Source: CAD feature listing. Evaluate the final solid. Frame: model axes, mm. A direction names the side the tool comes from. Give positions to 0.01 mm unless a question says otherwise; leave off trailing zeros. Loops run counter-clockwise (first coordinate to the right, second up) from the corner with the lowest first, then second, coordinate; pieces in that order, holes last. Notation, with made-up numbers: M -15,72 L 6,72 A24 cw 6,96 Z; hole C 58,-22 d9. An arc over 180 degrees is marked long. Answer in a Markdown table with one row per item.
```python
from build123d import *

# Parameters (mm, degrees)
SKETCH1_W           = 220
SKETCH1_H           = 130
BOSS_EXTRUDE1_DEPTH = 6
SKETCH2_W           = 90
SKETCH2_H           = 30
CUT_EXTRUDE1_DEPTH  = 128.910124697
FILLET1_R           = 15
SKETCH3_W           = 30
SKETCH3_H           = 6.2
BOSS_EXTRUDE2_DEPTH = 6


with BuildPart() as part:
    # Sketch1 → Boss-Extrude1 (new body)
    with BuildSketch(Plane(origin=(0, 0, 0), x_dir=(1, 0, 0), z_dir=(0, 1, 0))):
        Rectangle(SKETCH1_W, SKETCH1_H)
    extrude(amount=BOSS_EXTRUDE1_DEPTH)

    # Sketch2 → Cut-Extrude1 (cut, through all)
    with BuildSketch(Plane(origin=(0, 6, 0), x_dir=(1, 0, 0), z_dir=(0, 1, 0))):
        with Locations((-35, -50)):
            Rectangle(SKETCH2_W, SKETCH2_H)
        with Locations((-35, 50)):
            Rectangle(SKETCH2_W, SKETCH2_H)
    extrude(amount=-CUT_EXTRUDE1_DEPTH, mode=Mode.SUBTRACT)

    # Fillet1
    fillet1_edges = [part.edges().sort_by_distance(p)[0] for p in [
        (-80, 3, 35),
        (10, 3, 35),
        (-80, 3, -35),
        (10, 3, -35),
    ]]
    fillet(fillet1_edges, radius=FILLET1_R)

    # Sketch3 → Boss-Extrude2 (add)
    with BuildSketch(Plane(origin=(0, 6, 0), x_dir=(1, 0, 0), z_dir=(0, 1, 0))):
        with Locations((-95, 68.1)):
            Rectangle(SKETCH3_W, SKETCH3_H)
        with Locations((-95, -68.1)):
            Rectangle(SKETCH3_W, SKETCH3_H)
    extrude(amount=-BOSS_EXTRUDE2_DEPTH)


solid = part.part
```
Q1. Reachability of faces 1 (the flat face through (59, 3, 65)), 2 (the flat face through (-80, 3, 61)), 3 (the cylindrical face through (5.49, 2.96, -39.28)), 4 (the flat face through (59, 3, -65)) from +Z, -Z, +X, -X, +Y, -Y: full face, straight path, thin tool, end or side. Return the list, or none.
Values follow:
| item | result |
|---|---|
| face 1 | +Z, +X, +Y, -Y |
| face 2 | +Z, +Y, -Y |
| face 3 | -Z, +Y, -Y |
| face 4 | -Z, +X, +Y, -Y |
Q2. Contact query for flat-ended pins moving along their axis: pin 1 Ø1.8 at (x, y) = (45, 3.5) entering from +Z; pin 2 Ø1 at (x, y) = (36, 5) entering from -Z; pin 3 Ø1.8 at (x, y) = (-21.5, 2) entering from -Z. Output: stop coordinate, or through.
Values follow:
| item | result |
|---|---|
| pin 1 | z = 65 |
| pin 2 | z = -65 |
| pin 3 | z = -35 |
Q3. Section query C-C (x = 47.5). Output: boundary loops of the cut face in (y, z), plus the area to 3 significant figures.
Values follow:
| item | result |
|---|---|
| outline | M 0,-65 L 6,-65 L 6,65 L 0,65 Z |
| area | 780 mm^2 |
Q4. Section query D-D (x = -37). Output: boundary loops of the cut face in (y, z).
Values follow:
| item | result |
|---|---|
| outline | M 0,-35 L 6,-35 L 6,35 L 0,35 Z |
Q5. Section query B-B (z = 44.5). Output: boundary loops of the cut face in (x, y), plus the area to 3 significant figures.
Values follow:
| item | result |
|---|---|
| outline | M -110,0 L -78.96,0 L -78.96,6 L -110,6 Z; M 8.96,0 L 110,0 L 110,6 L 8.96,6 Z |
| area | 793 mm^2 |
Q6. Section query A-A (y = 3.95). Output: boundary loops of the cut face in (x, z).
Values follow:
| item | result |
|---|---|
| outline | M -110,-71.2 L -80,-71.2 L -80,-50 A15 cw -65,-35 L -5,-35 A15 cw 10,-50 L 10,-65 L 110,-65 L 110,65 L 10,65 L 10,50 A15 cw -5,35 L -65,35 A15 cw -80,50 L -80,71.2 L -110,71.2 Z |
Q7. Ray query, probe 1 along X at (y, z) = (0.3, -60); probe 2 along Z at (x, y) = (91.5, 0.75); probe 3 along Z at (x, y) = (-35.5, 2.3). Return the intervals inside material, ascending. Write a range as from..to.
Values follow:
| item | result |
|---|---|
| probe 1 | -110..-80, 10..110 |
| probe 2 | -65..65 |
| probe 3 | -35..35 |
